```python
from build123d import *

# Parameters (mm, degrees)
F0_W     = 15.58
F0_H     = 42.48
F1_DEPTH = 5
F3_DEPTH = 5
F5_DEPTH = 5
F6_R     = 1.5
F6_R_2   = 1
F7_DEPTH = 5
F9_DEPTH = 5


with BuildPart() as f1:
    # F0 (on Front) → F1 (new body)
    with BuildSketch(Plane.XZ):
        Rectangle(F0_W, F0_H)
    extrude(amount=-F1_DEPTH)

    # F2 (on face) → F3 (cut, through all)
    with BuildSketch(Plane.XZ):
        Polygon((4.91, 21.24), (7.79, 10.8), (7.79, 21.24), align=None)
    extrude(amount=-F3_DEPTH, mode=Mode.SUBTRACT)

    # F4 (on face) → F5 (cut, through all)
    with BuildSketch(Plane.XZ):
        Polygon((-2.19, -3.79), (-2.19, 21.24), (-7.79, 21.24), (-7.79, -12.515), align=None)
    extrude(amount=-F5_DEPTH, mode=Mode.SUBTRACT)

    # F6 (on face) → F7 (cut, through all)
    with BuildSketch(Plane.XZ):
        with Locations((3.75, 1.19)):
            Circle(F6_R)
        with Locations((3.17, 5.23)):
            Circle(F6_R_2)
        with Locations((2.23, 12.18)):
            Circle(F6_R_2)
        with Locations((1.68, 16.1)):
            Circle(F6_R)
    extrude(amount=-F7_DEPTH, mode=Mode.SUBTRACT)

    # F8 (on face) → F9 (cut, through all)
    with BuildSketch(Plane.XZ):
        with BuildLine():
            ThreePointArc((-1.21, -16.24), (-2.71, -17.74), (-1.21, -19.24))
            Line((-1.21, -19.24), (-1.21, -17.74))
            Line((-1.21, -17.74), (-1.21, -16.74))
            Line((-1.21, -16.74), (-1.21, -16.24))
        make_face()
        with BuildLine():
            Line((-1.21, -17.74), (-1.21, -19.24))
            ThreePointArc((-1.21, -19.24), (5.79, -12.24), (-1.21, -5.24))
            Line((-1.21, -5.24), (-1.21, -6.74))
            Line((-1.21, -6.74), (-1.21, -8.24))
            ThreePointArc((-1.21, -8.24), (2.79, -12.24), (-1.21, -16.24))
            Line((-1.21, -16.24), (-1.21, -16.74))
            Line((-1.21, -16.74), (-1.21, -17.74))
        make_face()
        with BuildLine():
            ThreePointArc((0.29, -12.24), (-2.27066, -11.17934), (-1.21, -13.74))
            ThreePointArc((-1.21, -13.74), (-0.14934, -13.30066), (0.29, -12.24))
        make_face()
        with BuildLine():
            Line((-1.21, -6.74), (-1.21, -5.24))
            ThreePointArc((-1.21, -5.24), (-2.71, -6.74), (-1.21, -8.24))
            Line((-1.21, -8.24), (-1.21, -6.74))
        make_face()
    extrude(amount=-F9_DEPTH, mode=Mode.SUBTRACT)


solid = f1.part
```
Part model, mm, in its own coordinate system. A direction names the side the tool comes from. Give positions to 0.01 mm unless a question says otherwise; leave off trailing zeros. Order: outer loops, then holes, each group sorted by start corner. A loop starts at its lowest first (then second) coordinate and runs counter-clockwise, first axis right, second up. Notation, with made-up numbers: (19.25, 79.25) - (76.25, 79.25) arc R12 ccw to (76.25, 93.25) - close; hole circle Ø8 at (75.5, -4). An arc over 180 degrees is marked (long way). Use one line per item in the form item = value.
Item 1: Two-plate mould, pull along X, no slides. Class faces 1 (the face through (5.136, 2.465, 0.615)), 2 (the face through (0, 2, -21.24)), 3 (the face through (-5.029, 2.465, -8.214)), 4 (the face through (2.79, 2.46, -12.15)): released by +X, released by -X, zero draft, split by the parting line, or undercut.
Solution:
face_1 = undercut
face_2 = zero draft
face_3 = released by -X
face_4 = undercut
Item 2: Slice it at C-C on z = 17. Give the cut face in (x, y), and give its area (3 significant figures).
Solution:
outline = (-2.19, 0) - (0.48, 0) - (0.48, 5) - (-2.19, 5) - close; (2.88, 0) - (6.08, 0) - (6.08, 5) - (2.88, 5) - close
area = 29.3 mm2
Item 3: Probe probe 1 along Z at (x, y) = (3.75, 1.9); probe 2 along Z at (x, y) = (1.68, 1.45); probe 3 along Z at (x, y) = (-2.5, 0.9). List the from-to ranges inside material, lowest first. Write a range as from..to.
Solution:
probe_1 = -21.24..-17.18, -7.3..-0.31, 2.69..4.42, 6.04..21.24
probe_2 = -21.24..-18.62, -15.01..-9.47, -5.86..11.34, 13.02..14.6, 17.6..21.24
probe_3 = -21.24..-18.51, -16.97..-13.01, -11.47..-7.51, -5.97..-4.27
Item 4: Slice it at D-D on x = 6.75. Give the cut face in (y, z), and give its area (3 significant figures).
Solution:
outline = (0, -21.24) - (5, -21.24) - (5, 14.57) - (0, 14.57) - close
area = 179 mm2
Item 5: Pin check, flat tips, straight feed: pin 1 Ø2.5 at (y, z) = (2, 5.5) entering from -X; pin 2 Ø1 at (x, z) = (-3.5, 2) entering from +Y; pin 3 Ø2 at (y, z) = (4, -3) entering from -X. Stop position of each tip, or through.
Solution:
pin_1 = -2.19
pin_2 = through
pin_3 = -2.32
Item 6: Slice it at B-B on y = 4.4. Give the cut face in (x, z) (3 decimals), and give its area (3 significant figures).
Solution:
outline = (-7.79, -21.24) - (7.79, -21.24) - (7.79, 10.8) - (4.91, 21.24) - (-2.19, 21.24) - (-2.19, -3.79) - (-7.79, -12.515) - close; hole circle Ø3 at (-1.21, -12.24); hole (-1.21, -19.24) arc R7 ccw to (-1.21, -5.24) arc R1.5 ccw to (-1.21, -8.24) arc R4 cw to (-1.21, -16.24) arc R1.5 ccw to start; hole circle Ø3 at (1.68, 16.1); hole circle Ø2 at (2.23, 12.18); hole circle Ø2 at (3.17, 5.23); hole circle Ø3 at (3.75, 1.19)
area = 396 mm2
Item 7: Which spindle directions (+Z, -Z, +X, -X, +Y, -Y) get a long thin tool onto all of the face, cutting with end or side? Do faces 5 (the face through (-2.71, 2.46, -6.71)), 6 (the face through (-2.19, 2, 9)), 7 (the face through (6.33, 2.46, 16.09)). Say none if no direction does.
Solution:
face_5 = +Y, -Y
face_6 = +Z, -X, +Y, -Y
face_7 = +Z, +X, +Y, -Y
Item 8: Slice it at A-A on z = 1.19. Give the cut face in (x, y).
Solution:
outline = (-2.19, 0) - (2.25, 0) - (2.25, 5) - (-2.19, 5) - close; (5.25, 0) - (7.79, 0) - (7.79, 5) - (5.25, 5) - close
